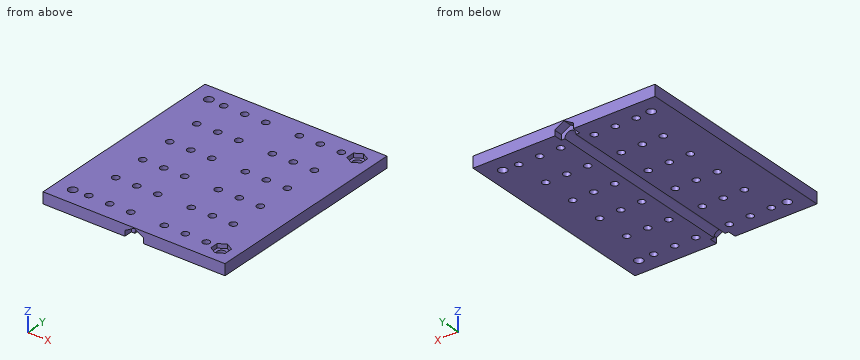
from build123d import *

# Parameters (mm, degrees)
F0_W     = 130
F0_H     = 150
F0_R     = 3.1
F0_R_2   = 2.5
F1_DEPTH = 8
F2_START = 5
F2_DEPTH = 20
F4_DEPTH = 150.001
F5_DEPTH = 6


# Not quite as in the source:
# - a pattern or mirror of a feature is missing from the dataset's text; its kind, count and spacing are read off the source's solid


with BuildPart() as f1:
    # F0 (on Top) → F1 (new body)
    with BuildSketch(Plane.XY):
        Rectangle(F0_W, F0_H)
        with Locations((-53, -63)):
            Circle(F0_R, mode=Mode.SUBTRACT)
        with Locations((-42, -62.5)):
            Circle(F0_R_2, mode=Mode.SUBTRACT)
        with Locations((-27, -62.5)):
            Circle(F0_R_2, mode=Mode.SUBTRACT)
        with Locations((-12, -62.5)):
            Circle(F0_R_2, mode=Mode.SUBTRACT)
        with Locations((-42, -37.5)):
            Circle(F0_R_2, mode=Mode.SUBTRACT)
        with Locations((-42, -12.5)):
            Circle(F0_R_2, mode=Mode.SUBTRACT)
        with Locations((-27, -37.5)):
            Circle(F0_R_2, mode=Mode.SUBTRACT)
        with Locations((-12, -37.5)):
            Circle(F0_R_2, mode=Mode.SUBTRACT)
        with Locations((-27, -12.5)):
            Circle(F0_R_2, mode=Mode.SUBTRACT)
        with Locations((-12, -12.5)):
            Circle(F0_R_2, mode=Mode.SUBTRACT)
        with Locations((12, -62.5)):
            Circle(F0_R_2, mode=Mode.SUBTRACT)
        with Locations((27, -62.5)):
            Circle(F0_R_2, mode=Mode.SUBTRACT)
        with Locations((42, -62.5)):
            Circle(F0_R_2, mode=Mode.SUBTRACT)
        Polygon((53, -57.1110272543), (58.1, -60.0555136271), (58.1, -65.9444863729), (53, -68.8889727457), (47.9, -65.9444863729), (47.9, -60.0555136271), align=None, mode=Mode.SUBTRACT)
        with Locations((12, -37.5)):
            Circle(F0_R_2, mode=Mode.SUBTRACT)
        with Locations((27, -37.5)):
            Circle(F0_R_2, mode=Mode.SUBTRACT)
        with Locations((12, -12.5)):
            Circle(F0_R_2, mode=Mode.SUBTRACT)
        with Locations((27, -12.5)):
            Circle(F0_R_2, mode=Mode.SUBTRACT)
        with Locations((42, -37.5)):
            Circle(F0_R_2, mode=Mode.SUBTRACT)
        with Locations((42, -12.5)):
            Circle(F0_R_2, mode=Mode.SUBTRACT)
        with Locations((-42, 12.5)):
            Circle(F0_R_2, mode=Mode.SUBTRACT)
        with Locations((-27, 12.5)):
            Circle(F0_R_2, mode=Mode.SUBTRACT)
        with Locations((-12, 12.5)):
            Circle(F0_R_2, mode=Mode.SUBTRACT)
        with Locations((-42, 37.5)):
            Circle(F0_R_2, mode=Mode.SUBTRACT)
        with Locations((-53, 63)):
            Circle(F0_R, mode=Mode.SUBTRACT)
        with Locations((-42, 62.5)):
            Circle(F0_R_2, mode=Mode.SUBTRACT)
        with Locations((-27, 37.5)):
            Circle(F0_R_2, mode=Mode.SUBTRACT)
        with Locations((-12, 37.5)):
            Circle(F0_R_2, mode=Mode.SUBTRACT)
        with Locations((-27, 62.5)):
            Circle(F0_R_2, mode=Mode.SUBTRACT)
        with Locations((-12, 62.5)):
            Circle(F0_R_2, mode=Mode.SUBTRACT)
        with Locations((12, 12.5)):
            Circle(F0_R_2, mode=Mode.SUBTRACT)
        with Locations((27, 12.5)):
            Circle(F0_R_2, mode=Mode.SUBTRACT)
        with Locations((42, 12.5)):
            Circle(F0_R_2, mode=Mode.SUBTRACT)
        with Locations((12, 37.5)):
            Circle(F0_R_2, mode=Mode.SUBTRACT)
        with Locations((27, 37.5)):
            Circle(F0_R_2, mode=Mode.SUBTRACT)
        with Locations((12, 62.5)):
            Circle(F0_R_2, mode=Mode.SUBTRACT)
        with Locations((27, 62.5)):
            Circle(F0_R_2, mode=Mode.SUBTRACT)
        with Locations((42, 37.5)):
            Circle(F0_R_2, mode=Mode.SUBTRACT)
        with Locations((42, 62.5)):
            Circle(F0_R_2, mode=Mode.SUBTRACT)
        Polygon((58.1, 65.9444863729), (58.1, 60.0555136271), (53, 57.1110272543), (47.9, 60.0555136271), (47.9, 65.9444863729), (53, 68.8889727457), align=None, mode=Mode.SUBTRACT)
        Polygon((53, 57.1110272543), (58.1, 60.0555136271), (58.1, 65.9444863729), (53, 68.8889727457), (47.9, 65.9444863729), (47.9, 60.0555136271), align=None)
        with Locations((53, 63)):
            Circle(F0_R, mode=Mode.SUBTRACT)
        Polygon((58.1, -65.9444863729), (58.1, -60.0555136271), (53, -57.1110272543), (47.9, -60.0555136271), (47.9, -65.9444863729), (53, -68.8889727457), align=None)
        with Locations((53, -63)):
            Circle(F0_R, mode=Mode.SUBTRACT)
    extrude(amount=F1_DEPTH)

    # F0 (on Top) → F2 (cut)
    with BuildSketch(Plane.XY.offset(F2_START)):
        Polygon((53, 57.1110272543), (58.1, 60.0555136271), (58.1, 65.9444863729), (53, 68.8889727457), (47.9, 65.9444863729), (47.9, 60.0555136271), align=None)
        with Locations((53, 63)):
            Circle(F0_R, mode=Mode.SUBTRACT)
        Polygon((58.1, -65.9444863729), (58.1, -60.0555136271), (53, -57.1110272543), (47.9, -60.0555136271), (47.9, -65.9444863729), (53, -68.8889727457), align=None)
        with Locations((53, -63)):
            Circle(F0_R, mode=Mode.SUBTRACT)
    extrude(amount=F2_DEPTH, mode=Mode.SUBTRACT)

    # F3 (on face) → F4 (cut, through all)
    with BuildSketch(Plane.XZ.offset(75)):
        with BuildLine():
            Line((-4, 0), (4, 0))
            ThreePointArc((4, 0), (0, 4), (-4, 0))
        make_face()
    extrude(amount=-F4_DEPTH, mode=Mode.SUBTRACT)

    # F3 (on face) → F5 (cut)
    with BuildSketch(Plane.XZ.offset(75)):
        with BuildLine():
            Line((6.6, 0), (4, 0))
            ThreePointArc((4, 0), (0, -4), (-4, 0))
            Line((-4, 0), (-6.6, 0))
            Line((-6.6, 0), (-6.6, -3.8105117767))
            Line((-6.6, -3.8105117767), (0, -7.6210235533))
            Line((0, -7.6210235533), (6.6, -3.8105117767))
            Line((6.6, -3.8105117767), (6.6, 0))
        make_face()
        with BuildLine():
            ThreePointArc((-4, 0), (0, 4), (4, 0))
            Line((4, 0), (6.6, 0))
            Line((6.6, 0), (6.6, 3.8105117767))
            Line((6.6, 3.8105117767), (0, 7.6210235533))
            Line((0, 7.6210235533), (-6.6, 3.8105117767))
            Line((-6.6, 3.8105117767), (-6.6, 0))
            Line((-6.6, 0), (-4, 0))
        make_face()
    f5 = extrude(amount=-F5_DEPTH, mode=Mode.SUBTRACT)

    # F5_copies: F5 across plane
    add(f5.mirror(Plane.ZX), mode=Mode.SUBTRACT)


solid = f1.part
Work out the finished part from the listing and answer in its coordinate system (mm). Coordinates: 2 decimals unless noted, no trailing zeros. Write each loop counter-clockwise with the first axis right and the second up, starting at its lowest first coordinate (ties: lowest second). Pieces come first, ordered by that corner, then holes. Notation, with made-up numbers: M 1,27.5 L 59,27.5 A26 ccw 59,66.5 Z; hole C 47,82.25 d7. An arc over 180 degrees is marked long. Use one line per item in the form item = value. Start each with the question number.
1. Straight lines are drawn through the part: probe 1 along Y at (x, z) = (-55.5, 5.5); probe 2 along Z at (x, y) = (48, -63); probe 3 along X at (y, z) = (3, 3). For each, find the intervals that lie inside material, in ascending order. Write a range as from..to.
2. The part is cut by section A-A (y = 37.5). Give the number of separate pieces and of enclosed holes in the cut face, plus the area to 3 significant figures.
3. The part is cut by section B-B (x = 27). Give the vertices of the cut face in (y, z).
4. Each of these flat-tipped pins is pushed along its axis until it touches: P1, Ø4, axis at x = -27, y = -12.5, coming from the -Z side; P2, Ø6, axis at x = -27, y = 12.5, coming from the -Z side. Where does it stop, or does it pass through?
5. The part is cut by section C-C (y = -3). Give the vertices of the cut face in (x, z).
Evaluation:
q1.probe_1 = -75..-64.83, -61.17..61.17, 64.83..75
q1.probe_2 = 0..5
q1.probe_3 = -65..-2.65, 2.65..65
q2.separate_pieces = 7
q2.enclosed_holes = 0
q2.area = 775 mm^2
q3.outline = M -75,0 L -65,0 L -65,8 L -75,8 Z; M -60,0 L -40,0 L -40,8 L -60,8 Z; M -35,0 L -15,0 L -15,8 L -35,8 Z; M -10,0 L 10,0 L 10,8 L -10,8 Z; M 15,0 L 35,0 L 35,8 L 15,8 Z; M 40,0 L 60,0 L 60,8 L 40,8 Z; M 65,0 L 75,0 L 75,8 L 65,8 Z
q4.P1 = through
q4.P2 = 0
q5.outline = M -65,0 L -4,0 A4 cw 4,0 L 65,0 L 65,8 L -65,8 Z
